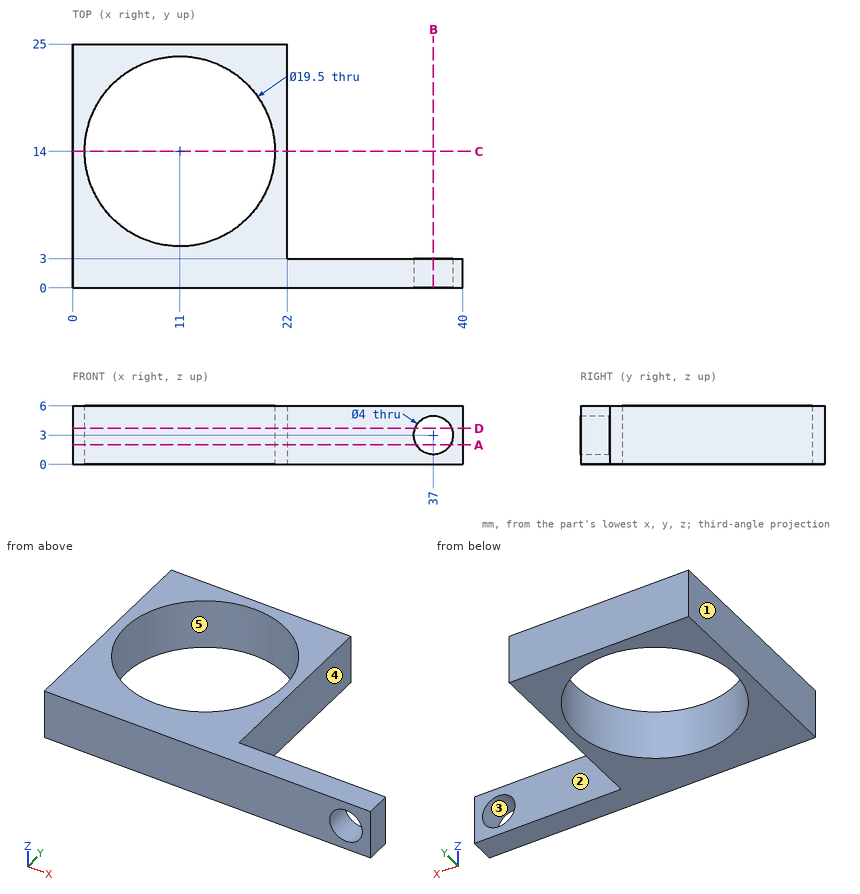
Could you check a few things on this drawing? It's one solid part, dimensions in mm from its lowest x, y, z. A direction names the side the tool comes from. Coordinates: 2 decimals unless noted, no trailing zeros. Write each loop counter-clockwise with the first axis right and the second up, starting at its lowest first coordinate (ties: lowest second). Pieces come first, ordered by that corner, then holes. Notation, with made-up numbers: (36.25, 24) - (82.25, 24) arc R18 cw to (82.25, 28) - close; hole circle Ø1 at (24, 59.25). An arc over 180 degrees is marked (long way). Return JSON: item names as keys, results as strings. Group by question number.
Item 1: Please list where these lines run through material, in increasing order: probe 1 along Y at (x, z) = (11, 3.1); probe 2 along X at (y, z) = (1.1, 3); probe 3 along Y at (x, z) = (25, 3.2).
Item 2: Which directions (+Z, -Z, +X, -X, +Y, -Y) give clear straight access to the entire face, cutting with the end or side of a thin tool? Please do the marked faces 4 and 5.
Item 3: If we section it at C-C (y = 14): Write out the boundary of the cut face in (x, z).
Item 4: If we section it at D-D (z = 3.7): Write out the boundary of the cut face in (x, y), then the cut area to 3 significant figures.
Item 5: If we section it at B-B (x = 37): Write out the boundary of the cut face in (y, z).
Item 6: We'd pull the mould along X, two halves only. Please class the marked faces 1, 2 and 3: pulls with the +X half, pulls with the -X half, needs draft (parallel to the pull), parting line crosses it, or undercut.
Item 7: If we section it at A-A (z = 2): Write out the boundary of the cut face in (x, y).
Item 8: I'm going to push flat-ended pins straight in: pin 1 Ø3 at (y, z) = (14, 4.5) entering from +X; pin 2 Ø3 at (x, z) = (27.5, 3.5) entering from +Y; pin 3 Ø1 at (x, y) = (23.5, 5.5) entering from -Z. Where does each tip first touch, or does it pass through?
Return value:
{
 "1": {"probe 1": "y = 0 to 4.25, 23.75 to 25", "probe 2": "x = 0 to 35, 39 to 40", "probe 3": "y = 0 to 3"},
 "2": {"face 4": "+Z, -Z, +X, +Y", "face 5": "+Z, -Z"},
 "3": {"outline": "(0, 0) - (1.25, 0) - (1.25, 6) - (0, 6) - close; (20.75, 0) - (22, 0) - (22, 6) - (20.75, 6) - close"},
 "4": {"outline": "(0, 0) - (35.13, 0) - (35.13, 3) - (22, 3) - (22, 25) - (0, 25) - close; (38.87, 0) - (40, 0) - (40, 3) - (38.87, 3) - close; hole circle Ø19.5 at (11, 14)", "area": "294 mm^2"},
 "5": {"outline": "(0, 0) - (3, 0) - (3, 1) - (0, 1) - close; (0, 5) - (3, 5) - (3, 6) - (0, 6) - close"},
 "6": {"face 1": "pulls with the -X half", "face 2": "needs draft", "face 3": "undercut"},
 "7": {"outline": "(0, 0) - (35.27, 0) - (35.27, 3) - (22, 3) - (22, 25) - (0, 25) - close; (38.73, 0) - (40, 0) - (40, 3) - (38.73, 3) - close; hole circle Ø19.5 at (11, 14)"},
 "8": {"pin 1": "stops at x = 22", "pin 2": "stops at y = 3", "pin 3": "passes through"}
}
